For this review, use the dimensioned drawing (mm, ordinates from the lowest corner) and the shaded views. Coordinates: 2 decimals unless noted, no trailing zeros. Loops run counter-clockwise (first coordinate to the right, second up) from the corner with the lowest first, then second, coordinate; pieces in that order, holes last.
1. To check wall thickness, follow probe 1 along Z at (x, y) = (32.5, 2.5); probe 2 along X at (y, z) = (5, 32.5). State the ranges of each line that lie inside material, in increasing order.
2. Take a section at A-A, the plane z = 57.5. State the section outline as (x, y) points.
3. Clearance check with flat-ended pins moving along their axes: P1, Ø4, axis at x = 23.57, z = 28.8, coming from the +Y side; P2, Ø5, axis at x = 58, z = 64, coming from the -Y side. State where each tip first meets the part, or that it passes through.
4. Take a section at B-B, the plane x = 7.5. State the section outline as (y, z) points, then the cut area to 3 significant figures.
5. Take a section at D-D, the plane z = 7.5. State the section outline as (x, y) points.
6. Take a section at C-C, the plane y = 2. Count the separate pieces of the cut face and the enclosed holes in it, then the cut area to 3 significant figures.
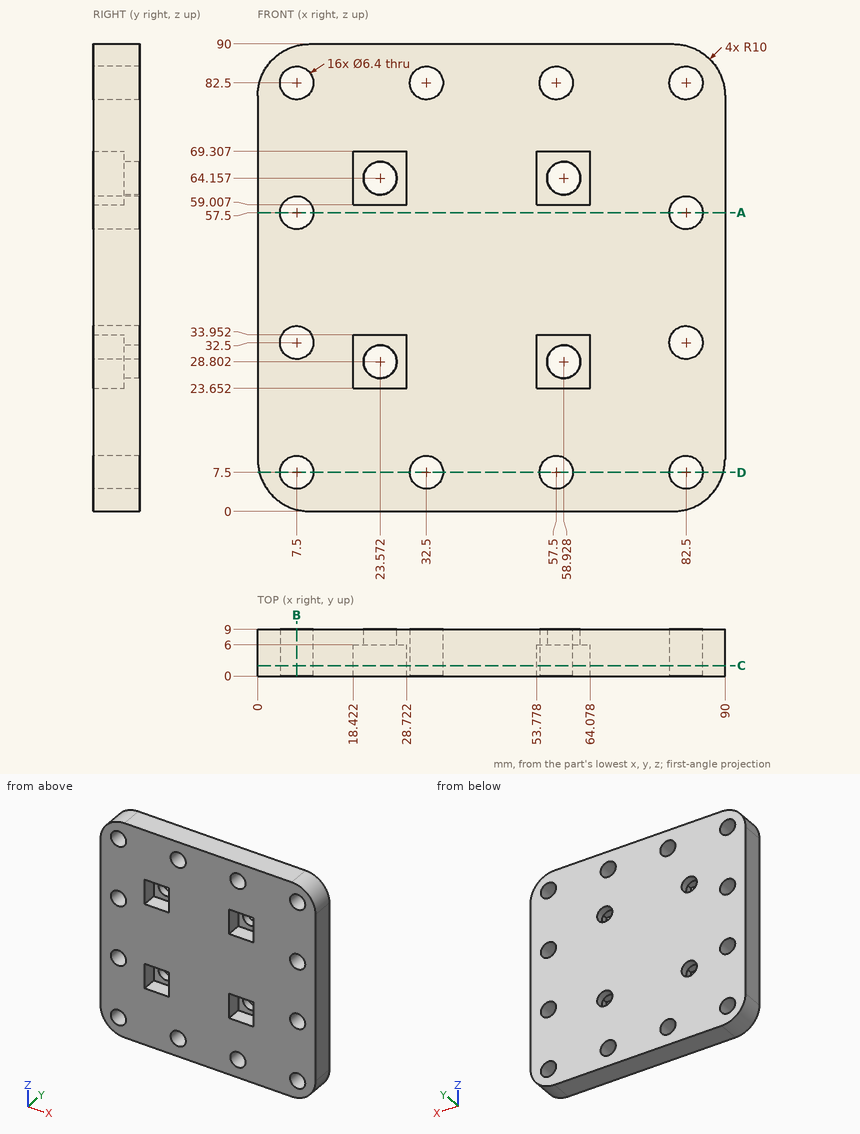
Results list:
1. probe 1: z = 0 to 4.3, 10.7 to 79.3, 85.7 to 90
1. probe 2: x = 0 to 4.3, 10.7 to 18.42, 28.72 to 53.78, 64.08 to 79.3, 85.7 to 90
2. outline: (0, 0) - (4.3, 0) - (4.3, 9) - (0, 9) - close; (10.7, 0) - (79.3, 0) - (79.3, 9) - (10.7, 9) - close; (85.7, 0) - (90, 0) - (90, 9) - (85.7, 9) - close
3. P1: passes through
3. P2: stops at y = 6
4. outline: (0, 0.32) - (9, 0.32) - (9, 4.3) - (0, 4.3) - close; (0, 10.7) - (9, 10.7) - (9, 29.3) - (0, 29.3) - close; (0, 35.7) - (9, 35.7) - (9, 54.3) - (0, 54.3) - close; (0, 60.7) - (9, 60.7) - (9, 79.3) - (0, 79.3) - close; (0, 85.7) - (9, 85.7) - (9, 89.68) - (0, 89.68) - close
4. area: 574 mm2
5. outline: (0.32, 0) - (4.3, 0) - (4.3, 9) - (0.32, 9) - close; (10.7, 0) - (29.3, 0) - (29.3, 9) - (10.7, 9) - close; (35.7, 0) - (54.3, 0) - (54.3, 9) - (35.7, 9) - close; (60.7, 0) - (79.3, 0) - (79.3, 9) - (60.7, 9) - close; (85.7, 0) - (89.68, 0) - (89.68, 9) - (85.7, 9) - close
6. separate pieces: 1
6. enclosed holes: 16
6. area: 7,200 mm2
